```python
from build123d import *

# Parameters (mm, degrees)
F1_DEPTH     = 10.16
F2_DEPTH     = 31.75
F3_DEPTH     = 38.1
F4_T1_DEPTH  = 182.2402005013
F4_T6_DEPTH  = 109.224523526
F4_T12_DEPTH = 109.224523526
F4_T18_DEPTH = 109.224523526
F4_T25_DEPTH = 109.224523526
F4_T31_DEPTH = 109.224523526
F4_T37_DEPTH = 109.224523526
F4_T43_DEPTH = 109.224523526
F4_T49_DEPTH = 109.224523526
F4_T56_DEPTH = 109.224523526
F4_T62_DEPTH = 109.224523526
F5_SIZE      = 3.81


# Not quite as in the source:
# - a fillet or chamfer that OpenCascade refuses, or shapes differently, is made with other operations: its cross-section is extruded or revolved along the edge and cut away or added


with BuildPart() as f1:
    # F0 (on Front) → F1 (new body, symmetric)
    with BuildSketch(Plane.XZ):
        with BuildLine():
            Line((59.4478547573, -51.4072924852), (42.545, 0))
            ThreePointArc((42.545, 0), (0, -42.545), (-42.545, 0))
            Line((-42.545, 0), (-59.4478547573, -51.4072924852))
            Line((-59.4478547573, -51.4072924852), (0, -51.4072924852))
            Line((0, -51.4072924852), (59.4478547573, -51.4072924852))
        make_face()
    extrude(amount=F1_DEPTH, both=True)

    # F0 (on Front) → F2 (join, symmetric)
    with BuildSketch(Plane.XZ):
        Polygon((0, -51.4072924852), (-59.4478547573, -51.4072924852), (-68.2578384876, -51.4072924852), (-68.2578384876, -66.9220536947), (0, -66.9220536947), align=None)
        Polygon((68.2578384876, -51.4072924852), (59.4478547573, -51.4072924852), (0, -51.4072924852), (0, -66.9220536947), (68.2578384876, -66.9220536947), align=None)
    extrude(amount=F2_DEPTH, both=True)

    # F0 (on Front) → F3 (join, symmetric)
    with BuildSketch(Plane.XZ):
        Polygon((74.3125453591, -66.9220536947), (68.2578384876, -66.9220536947), (0, -66.9220536947), (0, -71.3198781013), (74.3125453591, -71.3198781013), align=None)
        Polygon((0, -71.3198781013), (0, -66.9220536947), (-68.2578384876, -66.9220536947), (-74.3125453591, -66.9220536947), (-74.3125453591, -71.3198781013), align=None)
    extrude(amount=F3_DEPTH, both=True)

    # F4: chamfer of 8.89 on 4 edges, made by hand

    # F4_s2 → F4_t1 (cut)
    with BuildSketch(Plane.YZ.offset(-91.1201002506)):
        Polygon((-31.75, -60.2972924852), (-22.86, -51.4072924852), (-31.75, -51.4072924852), align=None)
        Polygon((31.75, -60.2972924852), (22.86, -51.4072924852), (31.75, -51.4072924852), align=None)
    extrude(amount=F4_T1_DEPTH, mode=Mode.SUBTRACT)


with BuildPart() as f4_tool4:
    # F4_s5 → F4_t6 (new body)
    with BuildSketch(Plane.XZ.offset(54.612261763)):
        Polygon((68.2578384876, -60.2972924852), (59.3678384876, -51.4072924852), (68.2578384876, -51.4072924852), align=None)
    extrude(amount=-F4_T6_DEPTH)

    split(bisect_by=Plane(origin=(38.3941614285, 0, 12.624102589), x_dir=(0, 1, 0), z_dir=(0.949966585, 0, 0.3123515446)), keep=Keep.TOP)

    split(bisect_by=Plane.XZ.offset(10.16), keep=Keep.TOP)


with BuildPart() as f1_1:
    add(f1.part)

    # F4_t3: cut F4_tool4
    add(f4_tool4.part, mode=Mode.SUBTRACT)


with BuildPart() as f4_tool10:
    # F4_s11 → F4_t12 (new body)
    with BuildSketch(Plane.XZ.offset(54.612261763)):
        Polygon((68.2578384876, -60.2972924852), (59.3678384876, -51.4072924852), (68.2578384876, -51.4072924852), align=None)
    extrude(amount=-F4_T12_DEPTH)

    split(bisect_by=Plane(origin=(38.3941614285, 0, 12.624102589), x_dir=(0, 1, 0), z_dir=(-0.949966585, 0, -0.3123515446)), keep=Keep.TOP)

    split(bisect_by=Plane.XZ.offset(10.16), keep=Keep.TOP)


with BuildPart() as f1_2:
    add(f1_1.part)

    # F4_t9: cut F4_tool10
    add(f4_tool10.part, mode=Mode.SUBTRACT)


with BuildPart() as f4_tool16:
    # F4_s17 → F4_t18 (new body)
    with BuildSketch(Plane.XZ.offset(54.612261763)):
        Polygon((68.2578384876, -60.2972924852), (59.3678384876, -51.4072924852), (68.2578384876, -51.4072924852), align=None)
    extrude(amount=-F4_T18_DEPTH)

    split(bisect_by=Plane(origin=(38.3941614285, 0, 12.624102589), x_dir=(0, 1, 0), z_dir=(0.949966585, 0, 0.3123515446)), keep=Keep.TOP)

    split(bisect_by=Plane.XZ.offset(-10.16), keep=Keep.TOP)

    split(bisect_by=Plane.XZ.offset(10.16), keep=Keep.BOTTOM)


with BuildPart() as f1_3:
    add(f1_2.part)

    # F4_t15: cut F4_tool16
    add(f4_tool16.part, mode=Mode.SUBTRACT)


with BuildPart() as f4_tool23:
    # F4_s24 → F4_t25 (new body)
    with BuildSketch(Plane.XZ.offset(54.612261763)):
        Polygon((68.2578384876, -60.2972924852), (59.3678384876, -51.4072924852), (68.2578384876, -51.4072924852), align=None)
    extrude(amount=-F4_T25_DEPTH)

    split(bisect_by=Plane(origin=(38.3941614285, 0, 12.624102589), x_dir=(0, 1, 0), z_dir=(0.949966585, 0, 0.3123515446)), keep=Keep.TOP)

    split(bisect_by=Plane.XZ.offset(-10.16), keep=Keep.BOTTOM)


with BuildPart() as f1_4:
    add(f1_3.part)

    # F4_t22: cut F4_tool23
    add(f4_tool23.part, mode=Mode.SUBTRACT)


with BuildPart() as f4_tool29:
    # F4_s30 → F4_t31 (new body)
    with BuildSketch(Plane.XZ.offset(54.612261763)):
        Polygon((68.2578384876, -60.2972924852), (59.3678384876, -51.4072924852), (68.2578384876, -51.4072924852), align=None)
    extrude(amount=-F4_T31_DEPTH)

    split(bisect_by=Plane(origin=(38.3941614285, 0, 12.624102589), x_dir=(0, 1, 0), z_dir=(-0.949966585, 0, -0.3123515446)), keep=Keep.TOP)

    split(bisect_by=Plane.XZ.offset(-10.16), keep=Keep.BOTTOM)


with BuildPart() as f1_5:
    add(f1_4.part)

    # F4_t28: cut F4_tool29
    add(f4_tool29.part, mode=Mode.SUBTRACT)


with BuildPart() as f4_tool35:
    # F4_s36 → F4_t37 (new body)
    with BuildSketch(Plane.XZ.offset(54.612261763)):
        Polygon((-68.2578384876, -60.2972924852), (-59.3678384876, -51.4072924852), (-68.2578384876, -51.4072924852), align=None)
    extrude(amount=-F4_T37_DEPTH)

    split(bisect_by=Plane(origin=(-38.3941614285, 0, 12.624102589), x_dir=(0, 1, 0), z_dir=(-0.949966585, 0, 0.3123515446)), keep=Keep.TOP)

    split(bisect_by=Plane.XZ.offset(10.16), keep=Keep.TOP)


with BuildPart() as f1_6:
    add(f1_5.part)

    # F4_t34: cut F4_tool35
    add(f4_tool35.part, mode=Mode.SUBTRACT)


with BuildPart() as f4_tool41:
    # F4_s42 → F4_t43 (new body)
    with BuildSketch(Plane.XZ.offset(54.612261763)):
        Polygon((-68.2578384876, -60.2972924852), (-59.3678384876, -51.4072924852), (-68.2578384876, -51.4072924852), align=None)
    extrude(amount=-F4_T43_DEPTH)

    split(bisect_by=Plane(origin=(-38.3941614285, 0, 12.624102589), x_dir=(0, 1, 0), z_dir=(0.949966585, 0, -0.3123515446)), keep=Keep.TOP)

    split(bisect_by=Plane.XZ.offset(10.16), keep=Keep.TOP)


with BuildPart() as f1_7:
    add(f1_6.part)

    # F4_t40: cut F4_tool41
    add(f4_tool41.part, mode=Mode.SUBTRACT)


with BuildPart() as f4_tool47:
    # F4_s48 → F4_t49 (new body)
    with BuildSketch(Plane.XZ.offset(54.612261763)):
        Polygon((-68.2578384876, -60.2972924852), (-59.3678384876, -51.4072924852), (-68.2578384876, -51.4072924852), align=None)
    extrude(amount=-F4_T49_DEPTH)

    split(bisect_by=Plane.XZ.offset(-10.16), keep=Keep.TOP)

    split(bisect_by=Plane(origin=(-38.3941614285, 0, 12.624102589), x_dir=(0, 1, 0), z_dir=(-0.949966585, 0, 0.3123515446)), keep=Keep.TOP)

    split(bisect_by=Plane.XZ.offset(10.16), keep=Keep.BOTTOM)


with BuildPart() as f1_8:
    add(f1_7.part)

    # F4_t46: cut F4_tool47
    add(f4_tool47.part, mode=Mode.SUBTRACT)


with BuildPart() as f4_tool54:
    # F4_s55 → F4_t56 (new body)
    with BuildSketch(Plane.XZ.offset(54.612261763)):
        Polygon((-68.2578384876, -60.2972924852), (-59.3678384876, -51.4072924852), (-68.2578384876, -51.4072924852), align=None)
    extrude(amount=-F4_T56_DEPTH)

    split(bisect_by=Plane.XZ.offset(-10.16), keep=Keep.BOTTOM)

    split(bisect_by=Plane(origin=(-38.3941614285, 0, 12.624102589), x_dir=(0, 1, 0), z_dir=(-0.949966585, 0, 0.3123515446)), keep=Keep.TOP)


with BuildPart() as f1_9:
    add(f1_8.part)

    # F4_t53: cut F4_tool54
    add(f4_tool54.part, mode=Mode.SUBTRACT)


with BuildPart() as f4_tool60:
    # F4_s61 → F4_t62 (new body)
    with BuildSketch(Plane.XZ.offset(54.612261763)):
        Polygon((-68.2578384876, -60.2972924852), (-59.3678384876, -51.4072924852), (-68.2578384876, -51.4072924852), align=None)
    extrude(amount=-F4_T62_DEPTH)

    split(bisect_by=Plane.XZ.offset(-10.16), keep=Keep.BOTTOM)

    split(bisect_by=Plane(origin=(-38.3941614285, 0, 12.624102589), x_dir=(0, 1, 0), z_dir=(0.949966585, 0, -0.3123515446)), keep=Keep.TOP)


with BuildPart() as f1_10:
    add(f1_9.part)

    # F4_t59: cut F4_tool60
    add(f4_tool60.part, mode=Mode.SUBTRACT)

    # F5
    f5_edges = [f1_10.edges().sort_by_distance(p)[0] for p in [
        (0, -38.1, -66.922054),
        (-74.312545, 0, -66.922054),
        (74.312545, 0, -66.922054),
        (0, 38.1, -66.922054),
    ]]
    chamfer(f5_edges, length=F5_SIZE)


solid = f1_10.part
```
Input: part model. Units: mm. Frame: model coordinates. A direction names the side the tool comes from. Round coordinates to 2 decimals unless told otherwise and drop trailing zeros. Loops run counter-clockwise (first coordinate to the right, second up) from the corner with the lowest first, then second, coordinate; pieces in that order, holes last.
1) Section query A-A on x = 0. Return the cut outline in (y, z) (3 decimals).
Ans:
outline: (-38.1, -71.32) - (38.1, -71.32) - (38.1, -70.732) - (34.29, -66.922) - (31.75, -66.922) - (31.75, -60.297) - (22.86, -51.407) - (10.16, -51.407) - (10.16, -42.545) - (-10.16, -42.545) - (-10.16, -51.407) - (-22.86, -51.407) - (-31.75, -60.297) - (-31.75, -66.922) - (-34.29, -66.922) - (-38.1, -70.732) - close
2) Set-up query: faces 1 (the flat face through (-1, -10.16, -43)), 2 (the flat face through (-68.258, 0, -64)), 3 (the flat face through (-1, 31.75, -64)), 4 (the flat face through (68.258, 0, -64)). Return all of +Z, -Z, +X, -X, +Y, -Y with unobstructed straight access to the full face (end or side cutting, diameter ignored); none if empty.
Ans:
face 1: +Z, +X, -X, -Y
face 2: +Z, -X, +Y, -Y
face 3: +Z, +X, -X, +Y
face 4: +Z, +X, +Y, -Y
3) Section query B-B on y = 17.5. Return the cut outline in (x, z).
Ans:
outline: (-74.31, -71.32) - (74.31, -71.32) - (74.31, -70.73) - (70.5, -66.92) - (68.26, -66.92) - (68.26, -60.3) - (59.37, -51.41) - (-59.37, -51.41) - (-68.26, -60.3) - (-68.26, -66.92) - (-70.5, -66.92) - (-74.31, -70.73) - close
4) Pin query (flat end, axial travel): pin 1 (2 mm diameter, centred on y = -14, z = -63.5, fed in from +X); pin 2 (15.5 mm diameter, centred on x = 19.5, z = -24.5, fed in from +Y); pin 3 (5.5 mm diameter, centred on x = 1.5, z = -63.5, fed in from +Y); pin 4 (6 mm diameter, centred on x = 58, z = -39.5, fed in from +Y). Return the tip coordinate at first contact, or that it passes through.
Ans:
pin 1: stops at x = 68.26
pin 2: passes through
pin 3: stops at y = 31.75
pin 4: stops at y = 10.16
5) Section query D-D on y = -1.5. Return the cut outline in (x, z) (1 decimal), plus the area to 3 significant figures.
Ans:
outline: (-74.3, -71.3) - (74.3, -71.3) - (74.3, -70.7) - (70.5, -66.9) - (68.3, -66.9) - (68.3, -60.3) - (59.5, -51.5) - (42.5, 0) arc R42.5 cw to (-42.5, 0) - (-59.5, -51.5) - (-68.3, -60.3) - (-68.3, -66.9) - (-70.5, -66.9) - (-74.3, -70.7) - close
area: 5,080 mm2
6) Material intervals for line 1 (Y direction, x = -37, z = -23); line 2 (Z direction, x = -15, y = 34); line 3 (Z direction, x = 54.5, y = -23), sorted ascending.
Ans:
line 1: y = -10.16 to 10.16
line 2: z = -71.32 to -66.92
line 3: z = -71.32 to -51.55
7) Section query C-C on z = -24. Return the cut outline in (x, y).
Ans:
outline: (-50.44, -10.16) - (-35.13, -10.16) - (-35.13, 10.16) - (-50.44, 10.16) - close; (35.13, -10.16) - (50.44, -10.16) - (50.44, 10.16) - (35.13, 10.16) - close
